For this review, take the finished solid that the model builds, in its own axes (mm). Face numbers are marked on the shaded views. A direction names the side the tool comes from. Coordinates: 2 decimals unless noted, no trailing zeros. Order: outer loops, then holes, each group sorted by start corner. A loop starts at its lowest first (then second) coordinate and runs counter-clockwise, first axis right, second up. Notation, with made-up numbers: M 33.25,4 L 50.25,4 A28 cw 50.25,37 Z; hole C -1.75,-33.75 d7. An arc over 180 degrees is marked long. Use CSV: the item, a comma, the result in double quotes.
```python
from build123d import *

# Parameters (mm, degrees)
F0_W         = 62.4540001154
F0_H         = 112.7128452063
F1_DEPTH     = 10
F3_R         = 11.8634694321
F4_DEPTH     = 25
F6_R         = 10.1380548027
F7_DEPTH     = 25
F9_SIZE      = 5
F10_T1_DEPTH = 133.4296750859
F10_T3_DEPTH = 88.1708299951


# Not quite as in the source:
# - a fillet or chamfer that OpenCascade refuses, or shapes differently, is made with other operations: its cross-section is extruded or revolved along the edge and cut away or added


with BuildPart() as f1:
    # F0 (on Top) → F1 (new body)
    with BuildSketch(Plane.XY):
        with Locations((31.2270000577, -6.0975924134)):
            Rectangle(F0_W, F0_H)
    extrude(amount=F1_DEPTH)

    # F3 (on face) → F4 (cut)
    with BuildSketch(Plane.XY.offset(10)):
        with Locations((31.0296863317, 29.0262252092)):
            Circle(F3_R)
    extrude(amount=-F4_DEPTH, mode=Mode.SUBTRACT)

    # F6 (on Top) → F7 (join)
    with BuildSketch(Plane.XY):
        with Locations((32.3501564562, -41.873395443)):
            Circle(F6_R)
    extrude(amount=F7_DEPTH)

    # F9
    f9_edges = [f1.edges().sort_by_distance(p)[0] for p in [
        (31.227, 50.25883, 10),
    ]]
    chamfer(f9_edges, length=F9_SIZE)

    # F10: chamfer of 5 on 5 edges, made by hand

    # F10_s2 → F10_t1 (cut)
    with BuildSketch(Plane.XZ.offset(-58.1172451295)):
        Polygon((57.4540001154, 10), (62.4540001154, 5), (62.4540001154, 10), align=None)
        Polygon((0, 5), (5, 10), (0, 10), align=None)
    extrude(amount=F10_T1_DEPTH, mode=Mode.SUBTRACT)

    # F10_s4 → F10_t3 (cut)
    with BuildSketch(Plane.YZ.offset(-12.8584149398)):
        Polygon((-57.4540150166, 10), (-62.4540150166, 5), (-62.4540150166, 10), align=None)
    extrude(amount=F10_T3_DEPTH, mode=Mode.SUBTRACT)

    # F10_s5 → F10_t6 (revolve, cut)
    with BuildSketch(Plane.XZ.offset(41.873395443)):
        Polygon((42.488211259, 20), (37.488211259, 25), (42.488211259, 25), align=None)
    revolve(axis=Axis((32.3501564562, -41.873395443, 25), (0, 0, 1)), mode=Mode.SUBTRACT)

    # F10_s7 → F10_t8 (revolve, cut)
    with BuildSketch(Plane.XZ.offset(-29.0262252092)):
        Polygon((47.8931557638, 10), (42.8931557638, 5), (42.8931557638, 10), align=None)
    revolve(axis=Axis((31.0296863317, 29.0262252092, 10), (0, 0, 1)), mode=Mode.SUBTRACT)


solid = f1.part
```
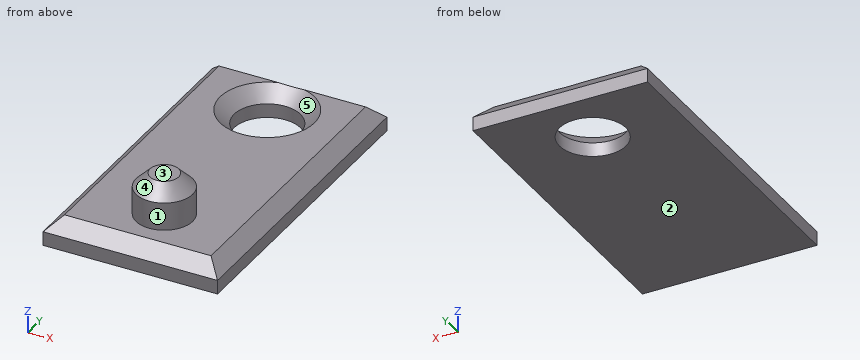
Item 1: Draft analysis for pull direction Y (two halves, no side actions). For the marked faces 3, 4 and 5, state which applies: released by +Y, released by -Y, zero draft, split by the parting line, or undercut.
Solutions:
face 3,"zero draft"
face 4,"split by the parting line"
face 5,"undercut"
Item 2: Add section D-D on z = 22.75. State the section outline as (x, y) points.
Solutions:
outline,"C 32.35,-41.87 d14.78"
Item 3: To check wall thickness, follow line 1 along Y through (x, z) = (35, 2.5); line 2 along Z through (x, y) = (52.5, 24.5); line 3 along X through (y, z) = (20, 6.75). State the ranges of each line that lie inside material, in increasing order. Write a range as [from, to].
Solutions:
line 1,"[-62.45, 17.85], [40.21, 50.26]"
line 2,"[0, 10]"
line 3,"[1.75, 20.84], [41.22, 60.7]"
Item 4: For the marked faces 1 and 2, list the 3-axis set-ups (+Z, -Z, +X, -X, +Y, -Y) from which the entire face can be reached by the end or side of a thin tool; tool diameter is ignored.
Solutions:
face 1,"+Z"
face 2,"-Z, +X, -X, +Y, -Y"
Item 5: Clearance check with flat-ended pins moving along their axes: pin 1 Ø1 at (x, y) = (10.5, 27.5) entering from +Z; pin 2 Ø4 at (y, z) = (-35, 15) entering from -X. State where each tip first meets the part, or that it passes through.
Solutions:
pin 1,"z = 10"
pin 2,"x = 23.46"
Item 6: Add section A-A on x = 51.5. State the section outline as (y, z) points.
Solutions:
outline,"M -62.45,0 L 50.26,0 L 50.26,5 L 45.26,10 L -57.45,10 L -62.45,5 Z"
Item 7: Add section C-C on z = 12. State the section outline as (x, y) points.
Solutions:
outline,"C 32.35,-41.87 d20.28"
Item 8: Add section B-B on y = -25.5. State the section outline as (x, z) points.
Solutions:
outline,"M 0,0 L 62.45,0 L 62.45,5 L 57.45,10 L 5,10 L 0,5 Z"
